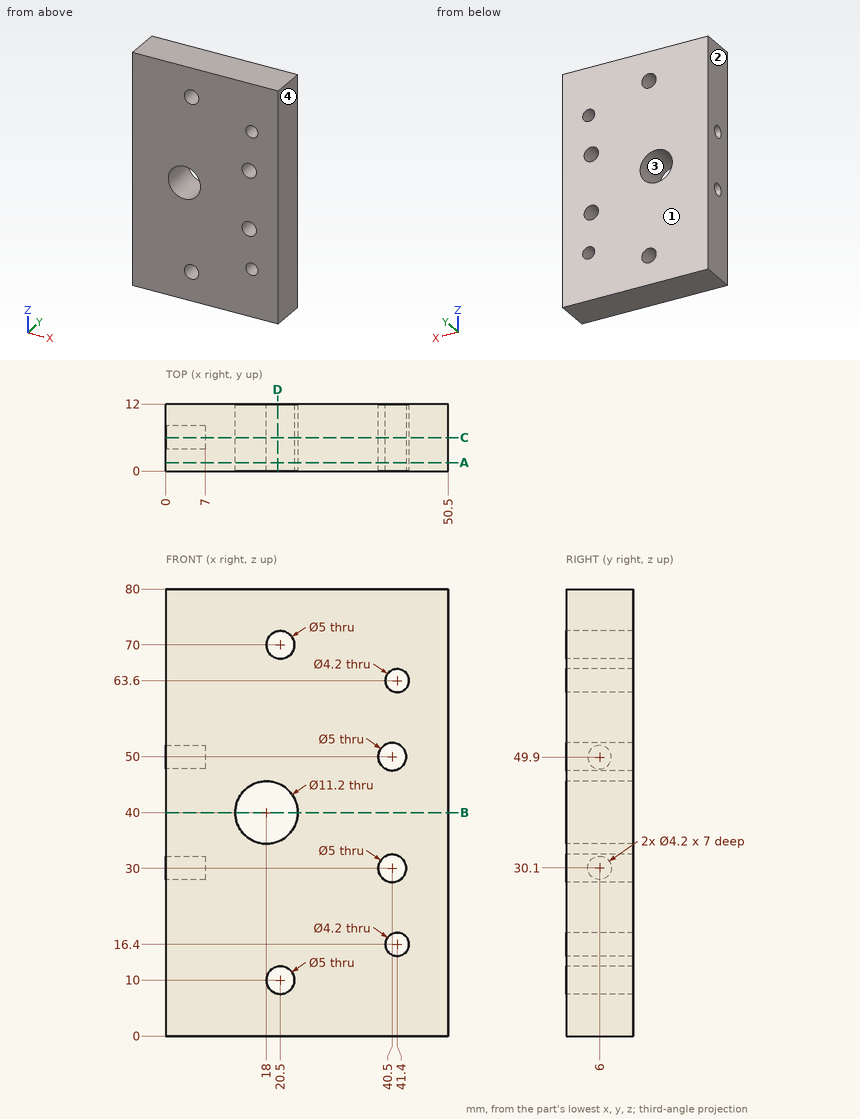
Job drawing, mm, ordinate dimensions from the low corner. One solid piece. Coordinates: 2 decimals unless noted, no trailing zeros. Order: outer loops, then holes, each group sorted by start corner. A loop starts at its lowest first (then second) coordinate and runs counter-clockwise, first axis right, second up. Notation, with made-up numbers: (6, 23.25) - (11, 23.25) arc R7 cw to (11, 28.25) - close; hole circle Ø5 at (-11, -23.5). An arc over 180 degrees is marked (long way). Return JSON: item names as keys, results as strings. Group by question number.
1) Flat gauge pin, fed straight in: P1, Ø2.5, axis at y = 6, z = 49.9, coming from the -X side. Where does the tip first touch, or does it go through?
2) Saw through at A-A, the plane y = 1.5. Write the cut outline in (x, z), plus the area to 3 significant figures.
3) Saw through at B-B, the plane z = 40. Write the cut outline in (x, y).
4) Saw through at C-C, the plane y = 6. Write the cut outline in (x, z), plus the area to 3 significant figures.
5) Probe line 1 (X direction, y = 8.75, z = 63.6); line 2 (Z direction, x = 40.5, y = 7); line 3 (X direction, y = 5.25, z = 70). List the from-to ranges inside material, lowest first. Write a range as from..to.
6) Saw through at D-D, the plane x = 20. Write the cut outline in (y, z).
7) Mould opens along X. For the marked faces 1, 2, 3 and 4 say: released by +X, released by -X, zero draft, split by the parting line, or undercut.
Values found:
{
 "1": {"P1": "stops at x = 7"},
 "2": {"outline": "(0, 0) - (50.5, 0) - (50.5, 80) - (0, 80) - close; hole circle Ø11.2 at (18, 40); hole circle Ø5 at (20.5, 10); hole circle Ø5 at (20.5, 70); hole circle Ø5 at (40.5, 30); hole circle Ø5 at (40.5, 50); hole circle Ø4.2 at (41.4, 16.4); hole circle Ø4.2 at (41.4, 63.6)", "area": "3,840 mm²"},
 "3": {"outline": "(0, 0) - (12.4, 0) - (12.4, 12) - (0, 12) - close; (23.6, 0) - (50.5, 0) - (50.5, 12) - (23.6, 12) - close"},
 "4": {"outline": "(0, 0) - (50.5, 0) - (50.5, 80) - (0, 80) - (0, 52) - (7, 52) - (7, 47.8) - (0, 47.8) - (0, 32.2) - (7, 32.2) - (7, 28) - (0, 28) - close; hole circle Ø11.2 at (18, 40); hole circle Ø5 at (20.5, 10); hole circle Ø5 at (20.5, 70); hole circle Ø5 at (40.5, 30); hole circle Ø5 at (40.5, 50); hole circle Ø4.2 at (41.4, 16.4); hole circle Ø4.2 at (41.4, 63.6)", "area": "3,780 mm²"},
 "5": {"line 1": "x = 0..39.3, 43.5..50.5", "line 2": "z = 0..14.5, 18.3..27.5, 32.5..47.5, 52.5..61.7, 65.5..80", "line 3": "x = 0..18, 23..50.5"},
 "6": {"outline": "(0, 0) - (12, 0) - (12, 7.55) - (0, 7.55) - close; (0, 12.45) - (12, 12.45) - (12, 34.77) - (0, 34.77) - close; (0, 45.23) - (12, 45.23) - (12, 67.55) - (0, 67.55) - close; (0, 72.45) - (12, 72.45) - (12, 80) - (0, 80) - close"},
 "7": {"face 1": "zero draft", "face 2": "released by -X", "face 3": "undercut", "face 4": "released by +X"}
}
